Input: part model. Units: mm. Frame: model coordinates. A direction names the side the tool comes from. Give positions to 0.01 mm unless a question says otherwise; leave off trailing zeros. Loops run counter-clockwise (first coordinate to the right, second up) from the corner with the lowest first, then second, coordinate; pieces in that order, holes last.
from build123d import *

# Parameters (mm, degrees)
SKETCH1_W                    = 39.878
SKETCH1_H                    = 50.8
BOSS_EXTRUDE1_DEPTH          = 73.025
CUT_EXTRUDE2_DEPTH           = 80.845941325
SKETCH9_R                    = 3.175
CUT_EXTRUDE4_DEPTH           = 87.994629196
CUT_SWEEP1_START             = 11.39698
CUT_SWEEP1_DEPTH             = 6.35
CUT_SWEEP1_START_2           = 55.27802
CUT_SWEEP1_2_DEPTH           = 6.35
F_10_0_1935_DIAMETER_HOLE1_D = 4.9149


# Read off the part's stored shape, not the designer's step: Cut-Sweep1
with BuildPart() as part:
    # Sketch1 → Boss-Extrude1 (new body)
    with BuildSketch(Plane(origin=(0, 0, 0), x_dir=(0, 0, -1), z_dir=(1, 0, 0))):
        Rectangle(SKETCH1_W, SKETCH1_H)
    extrude(amount=BOSS_EXTRUDE1_DEPTH)

    # Sketch3 → Cut-Extrude2 (cut, through all)
    with BuildSketch(Plane(origin=(73.025, 0, 0), x_dir=(0, 0, -1), z_dir=(1, 0, 0))):
        Polygon((6.35, 3.666174209), (0, 7.332348419), (-6.35, 3.666174209), (-6.35, -3.666174209), (0, -7.332348419), (6.35, -3.666174209), align=None)
    extrude(amount=-CUT_EXTRUDE2_DEPTH, mode=Mode.SUBTRACT)

    # Sketch9 → Cut-Extrude4 (cut, through all)
    with BuildSketch(Plane.XY.offset(19.939)):
        with Locations((9.525, 0)):
            Circle(SKETCH9_R)
        with Locations((36.5125, 0)):
            Circle(SKETCH9_R)
        with Locations((63.5, 0)):
            Circle(SKETCH9_R)
    extrude(amount=-CUT_EXTRUDE4_DEPTH, mode=Mode.SUBTRACT)

    # Cut-Sweep1 outline → Cut-Sweep1 (cut)
    with BuildSketch(Plane.YZ.offset(CUT_SWEEP1_START)):
        with BuildLine():
            add(Edge.make_bspline(
                [(-25.4, -15.1765), (-24.598155248, -15.176498148), (-23.769283214, -15.020738143), (-22.215051315, -14.383830521), (-21.491956074, -13.903011028), (-20.295262296, -12.697601351), (-19.822999045, -11.974685313), (-19.200412611, -10.432467289), (-19.050000001, -9.615195458), (-19.050000001, -8.8265)],
                knots=[0.025274121, 0.025274121, 0.025274121, 0.025274121, 0.088238261, 0.088238261, 0.1512024, 0.1512024, 0.214166539, 0.214166539, 0.277130679, 0.277130679, 0.277130679, 0.277130679], degree=3))
            Line((-25.4, -15.1765), (-25.4, -18.3515))
            add(Edge.make_bspline(
                [(-25.4, -18.3515), (-24.198801546, -18.351496292), (-22.962872636, -18.121523992), (-20.613629157, -17.158829003), (-19.544786623, -16.448168929), (-17.736040932, -14.626249639), (-17.037863537, -13.557113154), (-16.097253947, -11.227115749), (-15.875000001, -10.018094012), (-15.875000001, -8.8265)],
                knots=[0.025274121, 0.025274121, 0.025274121, 0.025274121, 0.088238261, 0.088238261, 0.1512024, 0.1512024, 0.214166539, 0.214166539, 0.277130679, 0.277130679, 0.277130679, 0.277130679], degree=3))
            Line((-15.875000001, -8.8265), (-15.875000001, 8.8265))
            add(Edge.make_bspline(
                [(-15.875000001, 8.8265), (-15.875000001, 10.154104999), (-16.148999917, 11.520161211), (-17.372865777, 14.155841649), (-18.276999964, 15.317491554), (-20.555768544, 17.157379798), (-21.841496853, 17.764411009), (-23.809992027, 18.242095131), (-24.446817823, 18.324942193), (-25.191458658, 18.349851774), (-25.29770495, 18.351585251), (-25.4, 18.351845725)],
                knots=[0.722867996, 0.722867996, 0.722867996, 0.722867996, 0.792150997, 0.792150997, 0.861433998, 0.861433998, 0.930716999, 0.930716999, 0.9653585, 0.9653585, 0.971358568, 0.971358568, 0.971358568, 0.971358568], degree=3))
            Line((-25.4, 18.351845725), (-25.4, 15.17649118))
            add(Edge.make_bspline(
                [(-19.050000001, 8.8265), (-19.050000001, 9.700178846), (-19.23785851, 10.633454764), (-20.043385287, 12.368213809), (-20.66121287, 13.161804707), (-22.160632803, 14.372442861), (-23.034678664, 14.786809878), (-24.336487637, 15.102712151), (-24.768983217, 15.158942974), (-25.259087559, 15.175338178), (-25.32981717, 15.176428808), (-25.4, 15.17649118)],
                knots=[0.722867996, 0.722867996, 0.722867996, 0.722867996, 0.792150997, 0.792150997, 0.861433998, 0.861433998, 0.930716999, 0.930716999, 0.9653585, 0.9653585, 0.971266218, 0.971266218, 0.971266218, 0.971266218], degree=3))
            Line((-19.050000001, 8.8265), (-19.050000001, -8.8265))
        make_face()
    extrude(amount=CUT_SWEEP1_DEPTH, mode=Mode.SUBTRACT)

    # Cut-Sweep1 2 outline → Cut-Sweep1 2 (cut)
    with BuildSketch(Plane.YZ.offset(CUT_SWEEP1_START_2)):
        with BuildLine():
            add(Edge.make_bspline(
                [(-25.4, -15.1765), (-24.598155248, -15.176498148), (-23.769283214, -15.020738143), (-22.215051315, -14.383830521), (-21.491956074, -13.903011028), (-20.295262296, -12.697601351), (-19.822999045, -11.974685313), (-19.200412611, -10.432467289), (-19.050000001, -9.615195458), (-19.050000001, -8.8265)],
                knots=[0.025274121, 0.025274121, 0.025274121, 0.025274121, 0.088238261, 0.088238261, 0.1512024, 0.1512024, 0.214166539, 0.214166539, 0.277130679, 0.277130679, 0.277130679, 0.277130679], degree=3))
            Line((-25.4, -15.1765), (-25.4, -18.3515))
            add(Edge.make_bspline(
                [(-25.4, -18.3515), (-24.198801546, -18.351496292), (-22.962872636, -18.121523992), (-20.613629157, -17.158829003), (-19.544786623, -16.448168929), (-17.736040932, -14.626249639), (-17.037863537, -13.557113154), (-16.097253947, -11.227115749), (-15.875000001, -10.018094012), (-15.875000001, -8.8265)],
                knots=[0.025274121, 0.025274121, 0.025274121, 0.025274121, 0.088238261, 0.088238261, 0.1512024, 0.1512024, 0.214166539, 0.214166539, 0.277130679, 0.277130679, 0.277130679, 0.277130679], degree=3))
            Line((-15.875000001, -8.8265), (-15.875000001, 8.8265))
            add(Edge.make_bspline(
                [(-15.875000001, 8.8265), (-15.875000001, 10.154104999), (-16.148999917, 11.520161211), (-17.372865777, 14.155841649), (-18.276999964, 15.317491554), (-20.555768544, 17.157379798), (-21.841496853, 17.764411009), (-23.809992027, 18.242095131), (-24.446817823, 18.324942193), (-25.191458658, 18.349851774), (-25.29770495, 18.351585251), (-25.4, 18.351845725)],
                knots=[0.722867996, 0.722867996, 0.722867996, 0.722867996, 0.792150997, 0.792150997, 0.861433998, 0.861433998, 0.930716999, 0.930716999, 0.9653585, 0.9653585, 0.971358568, 0.971358568, 0.971358568, 0.971358568], degree=3))
            Line((-25.4, 18.351845725), (-25.4, 15.17649118))
            add(Edge.make_bspline(
                [(-19.050000001, 8.8265), (-19.050000001, 9.700178846), (-19.23785851, 10.633454764), (-20.043385287, 12.368213809), (-20.66121287, 13.161804707), (-22.160632803, 14.372442861), (-23.034678664, 14.786809878), (-24.336487637, 15.102712151), (-24.768983217, 15.158942974), (-25.259087559, 15.175338178), (-25.32981717, 15.176428808), (-25.4, 15.17649118)],
                knots=[0.722867996, 0.722867996, 0.722867996, 0.722867996, 0.792150997, 0.792150997, 0.861433998, 0.861433998, 0.930716999, 0.930716999, 0.9653585, 0.9653585, 0.971266218, 0.971266218, 0.971266218, 0.971266218], degree=3))
            Line((-19.050000001, 8.8265), (-19.050000001, -8.8265))
        make_face()
    extrude(amount=CUT_SWEEP1_2_DEPTH, mode=Mode.SUBTRACT)

    # #10 (0.1935) Diameter Hole1 (through all)
    with Locations(Plane.XY.offset(19.939)):
        with Locations((9.525, 12.7), (36.5125, 12.7), (63.5, 12.7), (63.5, -12.7), (36.5125, -12.7), (9.525, -12.7)):
            Hole(F_10_0_1935_DIAMETER_HOLE1_D / 2)


solid = part.part
(1) Mould query, pull axis Y, two halves, no side actions, for faces 4 (the cylindrical face through (8.39, -14.88, -0.28)), 5 (the cylindrical face through (66.53, 0.95, -13.05)), 6 (the flat face through (36, 5, -19.939)), 7 (the flat face through (36, 25.4, 0)). Classes: +Y half, -Y half, draft (parallel to the pull), parting line (faces both ways), or undercut.
Values follow:
face 4: undercut
face 5: undercut
face 6: draft
face 7: +Y half
(2) Cut plane A-A (y = 12.7). Return the cut outline in (x, z) (3 decimals).
Values follow:
outline: (0, -19.939) - (7.068, -19.939) - (7.068, 19.939) - (0, 19.939) - close; (11.982, -19.939) - (34.055, -19.939) - (34.055, 19.939) - (11.982, 19.939) - close; (38.97, -19.939) - (61.043, -19.939) - (61.043, 19.939) - (38.97, 19.939) - close; (65.957, -19.939) - (73.025, -19.939) - (73.025, 19.939) - (65.957, 19.939) - close
(3) Cut plane C-C (y = 0). Count the separate pieces of the cut face and the enclosed holes in it, and give its area (3 significant figures).
Values follow:
separate pieces: 8
enclosed holes: 0
area: 1,470 mm2
(4) Cut plane B-B (x = 63.5). Return the cut outline in (y, z) (3 decimals), and give its area (3 significant figures).
Values follow:
outline: (-25.4, -19.939) - (-15.157, -19.939) - (-15.157, 19.939) - (-25.4, 19.939) - close; (-10.243, -19.939) - (-3.175, -19.939) - (-3.175, -6.35) - (-3.666, -6.35) - (-7.332, 0) - (-3.666, 6.35) - (-3.175, 6.35) - (-3.175, 19.939) - (-10.243, 19.939) - close; (3.175, -19.939) - (10.243, -19.939) - (10.243, 19.939) - (3.175, 19.939) - (3.175, 6.35) - (3.666, 6.35) - (7.332, 0) - (3.666, -6.35) - (3.175, -6.35) - close; (15.157, -19.939) - (25.4, -19.939) - (25.4, 19.939) - (15.157, 19.939) - close
area: 1,320 mm2
(5) Reachability of faces 1 (the flat face through (37, -3.3, -6.35)), 2 (the flat face through (11.397, -18, 0)), 3 (the cylindrical face through (65.45, -14.195, -0.279)) from +Z, -Z, +X, -X, +Y, -Y: full face, straight path, thin tool, end or side. Return the list, or none.
Values follow:
face 1: +X, -X
face 2: none
face 3: +Z, -Z
(6) Ray query, probe 1 along Y at (x, z) = (63.5, -15.5) (3 decimals); probe 2 along Y at (x, z) = (41.5, 0); probe 3 along Y at (x, z) = (63, -9). Return the intervals inside material, ascending.
Values follow:
probe 1: y = -25.4 to -15.157, -10.243 to -3.175, 3.175 to 10.243, 15.157 to 25.4
probe 2: y = -25.4 to -7.33, 7.33 to 25.4
probe 3: y = -25.4 to -15.11, -10.29 to -3.14, 3.14 to 10.29, 15.11 to 25.4
(7) Cut plane D-D (x = 24.5). Return the cut outline in (y, z).
Values follow:
outline: (-25.4, -19.94) - (25.4, -19.94) - (25.4, 19.94) - (-25.4, 19.94) - close; hole (-7.33, 0) - (-3.67, -6.35) - (3.67, -6.35) - (7.33, 0) - (3.67, 6.35) - (-3.67, 6.35) - close
